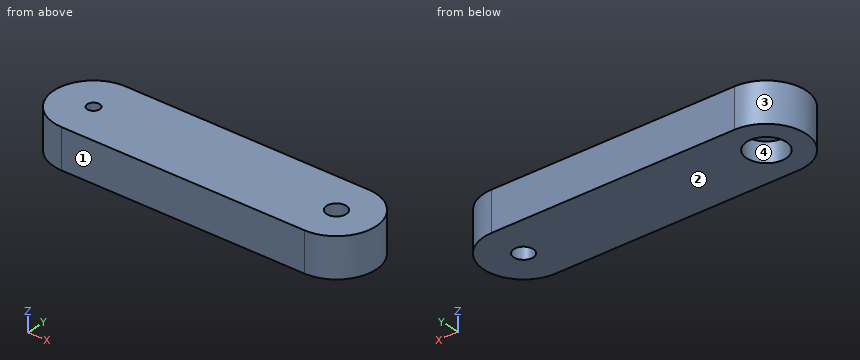
Autodesk Inventor part; units mm, degrees
ref_plane "YZ Plane" through (0, 0, 0) normal (1, 0, 0) x (0, 1, 0)
ref_plane "XZ Plane" through (0, 0, 0) normal (0, 1, 0) x (-1, 0, 0)
ref_plane "XY Plane" through (0, 0, 0) normal (0, 0, 1) x (1, 0, 0)
sketch "Sketch1" plane through (0, 0, 0) normal (0, 0, 1) x (1, 0, 0)
  line L0 (19.685, 0) -> (-19.685, 0) construction
  line L1 (19.685, 6.35) -> (-19.685, 6.35)
  line L2 (-19.685, -6.35) -> (19.685, -6.35)
  arc A0 (19.685, -6.35) -> (19.685, 6.35) centre (19.685, 0) ccw
  arc A1 (-19.685, 6.35) -> (-19.685, -6.35) centre (-19.685, 0) ccw
  circle A2 centre (-19.685, 0) radius 3.175
  circle A3 centre (19.685, 0) radius 1.5875
  point P0 (0, 0)
  dimension "d0" = 6.35
  dimension "d1" = 39.37
  dimension "d2" = 6.35
  dimension "d3" = 3.175
extrude "Extrusion1" add sketch "Sketch1" along normal blind 3.175
sketch "Sketch2" plane through (0, 0, 3.175) normal (0, 0, 1) x (1, 0, 0)
  arc A0 (-19.685, 6.35) -> (-19.685, -6.35) centre (-19.685, 0) ccw
  line L0 (-19.685, -6.35) -> (19.685, -6.35)
  arc A1 (19.685, -6.35) -> (19.685, 6.35) centre (19.685, 0) ccw
  line L1 (19.685, 6.35) -> (-19.685, 6.35)
  circle A2 centre (19.685, 0) radius 1.5875
  circle A3 centre (-19.685, 0) radius 3.175
  circle A4 centre (-19.685, 0) radius 1
  point P0 (0, 0)
  dimension "d6" = 2
extrude "Extrusion2" add sketch "Sketch2" along normal blind 3.175 contours L1 A1 L0 A0 | A3
properties part number "bunny neck"
Input: part model. Units: mm. Frame: model coordinates. Face numbers are marked on the shaded views. Give positions to 0.01 mm unless a question says otherwise; leave off trailing zeros. Order: outer loops, then holes, each group sorted by start corner. A loop starts at its lowest first (then second) coordinate and runs counter-clockwise, first axis right, second up.
1. Cut plane C-C (x = -17). Return loops of the section in (y, z) (3 decimals).
Computed:
outline: (-6.35, 0) - (-1.695, 0) - (-1.695, 3.175) - (1.695, 3.175) - (1.695, 0) - (6.35, 0) - (6.35, 6.35) - (-6.35, 6.35) - close
2. Line query: probe 1 along Z at (x, y) = (-21, 2) (3 decimals); probe 2 along X at (y, z) = (1.75, 2); probe 3 along Y at (x, z) = (20.5, 5.5). Output: solid intervals per line, ascending.
Computed:
probe 1: z = 3.175 to 6.35
probe 2: x = -25.79 to -22.33, -17.04 to 25.79
probe 3: y = -6.3 to -1.36, 1.36 to 6.3
3. Pin query (flat end, axial travel): pin 1 Ø3 at (x, y) = (-19.5, 1) entering from -Z (3 decimals); pin 2 Ø2 at (y, z) = (5, 0.5) entering from -X. Return the tip coordinate at first contact, or that it passes through.
Computed:
pin 1: stops at z = 3.175
pin 2: stops at x = -24.62
4. Cut plane A-A (y = 0). State how many separate pieces and enclosed holes the cut face has, and give its area (3 significant figures).
Computed:
separate pieces: 3
enclosed holes: 0
area: 284 mm2
5. Cut plane D-D (y = -2.25). Return loops of the section in (x, z) (3 decimals).
Computed:
outline: (-25.623, 0) - (-21.925, 0) - (-21.925, 3.175) - (-17.445, 3.175) - (-17.445, 0) - (25.623, 0) - (25.623, 6.35) - (-25.623, 6.35) - close
6. Draft query along Y for the marked faces 1, 2, 3 and 4. Return one class per face: released by +Y, released by -Y, zero draft, split by the parting line, or undercut.
Computed:
face 1: released by -Y
face 2: zero draft
face 3: split by the parting line
face 4: undercut
